```python
from build123d import *

# Parameters (mm, degrees)
SKETCH_1_W             = 60
SKETCH_1_H             = 652
EXTRUDE_1_DEPTH        = 3
SKETCH_2_R             = 1.65
CUT_EXTRUDE_1_DEPTH    = 3
FILLET_1_R             = 2
SKETCH_4_R             = 1.65
CUT_EXTRUDE_2_DEPTH    = 10
CUT_EXTRUDE_3_DEPTH    = 3
PATTERN_LINEAR_2_COUNT = 7
PATTERN_LINEAR_2_PITCH = 65
MIRROR_1_COPY_1_DEPTH  = 3
MIRROR_1_COPY_2_DEPTH  = 3
MIRROR_1_COPY_3_DEPTH  = 3
MIRROR_1_COPY_4_DEPTH  = 3
MIRROR_1_COPY_5_DEPTH  = 3
MIRROR_1_COPY_6_DEPTH  = 3
SKETCH_6_R             = 1.65
CUT_EXTRUDE_4_DEPTH    = 10


with BuildPart() as part:
    # 草图1 → 凸台-拉伸1 (new body)
    with BuildSketch(Plane(origin=(0, 0, 0), x_dir=(1, 0, 0), z_dir=(0, 1, 0))):
        Rectangle(SKETCH_1_W, SKETCH_1_H)
    extrude(amount=EXTRUDE_1_DEPTH)

    # 草图2 → 切除-拉伸1 (cut)
    with BuildSketch(Plane(origin=(0, 3, 0), x_dir=(1, 0, 0), z_dir=(0, 1, 0))):
        with Locations(Location((0, -306, 0), (0, 0, 270))):
            Circle(SKETCH_2_R)
        with Locations(Location((0, -236, 0), (0, 0, 270))):
            Circle(SKETCH_2_R)
        with Locations(Location((0, -184, 0), (0, 0, 270))):
            Circle(SKETCH_2_R)
        with Locations(Location((0, -159, 0), (0, 0, 270))):
            Circle(SKETCH_2_R)
        with Locations(Location((0, 316, 0), (0, 0, 270))):
            Circle(SKETCH_2_R)
        with Locations(Location((0, 291, 0), (0, 0, 270))):
            Circle(SKETCH_2_R)
        with Locations(Location((0, 266, 0), (0, 0, 270))):
            Circle(SKETCH_2_R)
        with Locations(Location((0, 241, 0), (0, 0, 270))):
            Circle(SKETCH_2_R)
    extrude(amount=-CUT_EXTRUDE_1_DEPTH, mode=Mode.SUBTRACT)

    # 圆角1
    fillet_1_edges = [part.edges().sort_by_distance(p)[0] for p in [
        (30, 1.5, 326),
        (-30, 1.5, 326),
        (-30, 1.5, -326),
        (30, 1.5, -326),
    ]]
    fillet(fillet_1_edges, radius=FILLET_1_R)

    # 草图4 → 切除-拉伸2 (cut)
    with BuildSketch(Plane(origin=(0, 3, 0), x_dir=(1, 0, 0), z_dir=(0, 1, 0))):
        with Locations(Location((20, -283, 0), (0, 0, 270))):
            Circle(SKETCH_4_R)
        with Locations(Location((-20, -283, 0), (0, 0, 270))):
            Circle(SKETCH_4_R)
    extrude(amount=-CUT_EXTRUDE_2_DEPTH, mode=Mode.SUBTRACT)

    # 草图5 → 切除-拉伸3 (cut)
    with BuildSketch(Plane(origin=(0, 3, 0), x_dir=(1, 0, 0), z_dir=(0, 1, 0))):
        with BuildLine():
            Line((14, -186), (14, -146))
            ThreePointArc((14, -146), (18, -142), (22, -146))
            Line((22, -146), (22, -186))
            ThreePointArc((22, -186), (18, -190), (14, -186))
        make_face()
    cut_extrude_3 = extrude(amount=-CUT_EXTRUDE_3_DEPTH, mode=Mode.SUBTRACT)

    # 阵列(线性)2: 切除-拉伸3 ×7
    with Locations(*[(0, 0, -i * PATTERN_LINEAR_2_PITCH) for i in range(1, PATTERN_LINEAR_2_COUNT)]):
        add(cut_extrude_3, mode=Mode.SUBTRACT)

    # 镜向1: 切除-拉伸3 across plane
    add(cut_extrude_3.mirror(Plane(origin=(0, 0, 0), x_dir=(0, 0, 1), z_dir=(1, 0, 0))), mode=Mode.SUBTRACT)

    # 镜向1 copy 1 sketch → 镜向1 copy 1 (cut)
    with BuildSketch(Plane(origin=(0, 3, -65), x_dir=(-1, 0, 0), z_dir=(0, 1, 0))):
        with BuildLine():
            Line((14, 186), (14, 146))
            ThreePointArc((14, 146), (18, 142), (22, 146))
            Line((22, 146), (22, 186))
            ThreePointArc((22, 186), (18, 190), (14, 186))
        make_face()
    extrude(amount=-MIRROR_1_COPY_1_DEPTH, mode=Mode.SUBTRACT)

    # 镜向1 copy 2 sketch → 镜向1 copy 2 (cut)
    with BuildSketch(Plane(origin=(0, 3, -130), x_dir=(-1, 0, 0), z_dir=(0, 1, 0))):
        with BuildLine():
            Line((14, 186), (14, 146))
            ThreePointArc((14, 146), (18, 142), (22, 146))
            Line((22, 146), (22, 186))
            ThreePointArc((22, 186), (18, 190), (14, 186))
        make_face()
    extrude(amount=-MIRROR_1_COPY_2_DEPTH, mode=Mode.SUBTRACT)

    # 镜向1 copy 3 sketch → 镜向1 copy 3 (cut)
    with BuildSketch(Plane(origin=(0, 3, -195), x_dir=(-1, 0, 0), z_dir=(0, 1, 0))):
        with BuildLine():
            Line((14, 186), (14, 146))
            ThreePointArc((14, 146), (18, 142), (22, 146))
            Line((22, 146), (22, 186))
            ThreePointArc((22, 186), (18, 190), (14, 186))
        make_face()
    extrude(amount=-MIRROR_1_COPY_3_DEPTH, mode=Mode.SUBTRACT)

    # 镜向1 copy 4 sketch → 镜向1 copy 4 (cut)
    with BuildSketch(Plane(origin=(0, 3, -260), x_dir=(-1, 0, 0), z_dir=(0, 1, 0))):
        with BuildLine():
            Line((14, 186), (14, 146))
            ThreePointArc((14, 146), (18, 142), (22, 146))
            Line((22, 146), (22, 186))
            ThreePointArc((22, 186), (18, 190), (14, 186))
        make_face()
    extrude(amount=-MIRROR_1_COPY_4_DEPTH, mode=Mode.SUBTRACT)

    # 镜向1 copy 5 sketch → 镜向1 copy 5 (cut)
    with BuildSketch(Plane(origin=(0, 3, -325), x_dir=(-1, 0, 0), z_dir=(0, 1, 0))):
        with BuildLine():
            Line((14, 186), (14, 146))
            ThreePointArc((14, 146), (18, 142), (22, 146))
            Line((22, 146), (22, 186))
            ThreePointArc((22, 186), (18, 190), (14, 186))
        make_face()
    extrude(amount=-MIRROR_1_COPY_5_DEPTH, mode=Mode.SUBTRACT)

    # 镜向1 copy 6 sketch → 镜向1 copy 6 (cut)
    with BuildSketch(Plane(origin=(0, 3, -390), x_dir=(-1, 0, 0), z_dir=(0, 1, 0))):
        with BuildLine():
            Line((14, 186), (14, 146))
            ThreePointArc((14, 146), (18, 142), (22, 146))
            Line((22, 146), (22, 186))
            ThreePointArc((22, 186), (18, 190), (14, 186))
        make_face()
    extrude(amount=-MIRROR_1_COPY_6_DEPTH, mode=Mode.SUBTRACT)

    # 草图6 → 切除-拉伸4 (cut)
    with BuildSketch(Plane.XZ):
        with Locations(Location((0, 254, 0), (0, 0, 270))):
            Circle(SKETCH_6_R)
        with Locations(Location((0, 214, 0), (0, 0, 270))):
            Circle(SKETCH_6_R)
    extrude(amount=-CUT_EXTRUDE_4_DEPTH, mode=Mode.SUBTRACT)


solid = part.part
```
Part model, mm, in its own coordinate system. Round coordinates to 2 decimals unless told otherwise and drop trailing zeros. Loops run counter-clockwise (first coordinate to the right, second up) from the corner with the lowest first, then second, coordinate; pieces in that order, holes last. Notation, with made-up numbers: (-15.75, -8) -> (26.25, -8) arc R13 ccw to (26.25, 1) -> close; hole circle Ø6 at (11, 55.25). An arc over 180 degrees is marked (long way). Use one line per item in the form item = value. Start each with the question number.
Item 1: Band-saw the part on A-A (z = -18.5). List the corners of the cut face in (x, y), plus the area to 3 significant figures.
Item 2: Band-saw the part on B-B (y = 2.2). Give the number of separate pieces and of enclosed holes in the cut face, plus the area to 3 significant figures.
Item 3: Drill centre lines: line 1 along X through (y, z) = (2.2, -241); line 2 along X through (y, z) = (2.4, -73); line 3 along X through (y, z) = (0.85, 100.5). Where is each one in solid material? Low to high.
Data:
q1.outline = (-30, 0) -> (-22, 0) -> (-22, 3) -> (-30, 3) -> close; (-14, 0) -> (14, 0) -> (14, 3) -> (-14, 3) -> close; (22, 0) -> (30, 0) -> (30, 3) -> (22, 3) -> close
q1.area = 132 mm^2
q2.separate_pieces = 1
q2.enclosed_holes = 26
q2.area = 33,800 mm^2
q3.line_1 = -30 to -22, -14 to -1.65, 1.65 to 14, 22 to 30
q3.line_2 = -30 to -21.87, -14.13 to 14.13, 21.87 to 30
q3.line_3 = -30 to -22, -14 to 14, 22 to 30
